from build123d import *

# Parameters (mm, degrees)
BOSS_EXTRUDE1_DEPTH                              = 2.3
BOSS_EXTRUDE2_START                              = 6.7
BOSS_EXTRUDE2_DEPTH                              = 6.7
BOSS_EXTRUDE3_DEPTH                              = 0.5
SKETCH4_R                                        = 12.925
BOSS_EXTRUDE4_DEPTH                              = 7.6
DRAFT1_ANGLE                                     = 56.309932527
DRAFT2_ANGLE                                     = 56.309932527
DRAFT3_ANGLE                                     = 56.309932527
DRAFT4_ANGLE                                     = 56.309932527
SKETCH5_R                                        = 8.025
CUT_EXTRUDE1_DEPTH                               = 8
CUT_EXTRUDE2_DEPTH                               = 1.65
CBORE_FOR_M8_HEX_HEAD_BOLT1_D                    = 9.25
CBORE_FOR_M8_HEX_HEAD_BOLT1_CBORE_D              = 12
CBORE_FOR_M8_HEX_HEAD_BOLT1_CBORE_DEPTH          = 0.65
CBORE_FOR_M3_HEX_HEAD_MACHINE_SCREW1_D           = 3.5
CBORE_FOR_M3_HEX_HEAD_MACHINE_SCREW1_DEPTH       = 9.9
CBORE_FOR_M3_HEX_HEAD_MACHINE_SCREW1_CBORE_D     = 6
CBORE_FOR_M3_HEX_HEAD_MACHINE_SCREW1_CBORE_DEPTH = 2.45
CHAMFER1_SIZE                                    = 0.25
CHAMFER4_SIZE                                    = 0.5
CHAMFER4_SIZE2                                   = 0.9
FILLET1_R                                        = 0.150000001
FILLET2_R                                        = 0.499999999


with BuildPart() as part:
    # Sketch1 → Boss-Extrude1 (new body)
    with BuildSketch(Plane.XZ.offset(-6.7)):
        with BuildLine():
            Line((8.625, -20.875), (16.316766683, -20.875))
            ThreePointArc((16.316766683, -20.875), (17.01460187, -20.749306819), (17.624723932, -20.388026052))
            ThreePointArc((17.624723932, -20.388026052), (19.056527753, -19.056527753), (20.388026052, -17.624723932))
            ThreePointArc((20.388026052, -17.624723932), (20.749306819, -17.01460187), (20.875, -16.316766683))
            Line((20.875, -16.316766683), (20.875, 16.316766683))
            ThreePointArc((20.875, 16.316766683), (20.749306819, 17.01460187), (20.388026052, 17.624723932))
            ThreePointArc((20.388026052, 17.624723932), (19.056527753, 19.056527753), (17.624723932, 20.388026052))
            ThreePointArc((17.624723932, 20.388026052), (17.01460187, 20.749306819), (16.316766683, 20.875))
            Line((16.316766683, 20.875), (-16.316766683, 20.875))
            ThreePointArc((-16.316766683, 20.875), (-17.01460187, 20.749306819), (-17.624723932, 20.388026052))
            ThreePointArc((-17.624723932, 20.388026052), (-19.056527753, 19.056527753), (-20.388026052, 17.624723932))
            ThreePointArc((-20.388026052, 17.624723932), (-20.749306819, 17.01460187), (-20.875, 16.316766683))
            Line((-20.875, 16.316766683), (-20.875, -16.316766683))
            ThreePointArc((-20.875, -16.316766683), (-20.749306819, -17.01460187), (-20.388026052, -17.624723932))
            ThreePointArc((-20.388026052, -17.624723932), (-19.056527753, -19.056527753), (-17.624723932, -20.388026052))
            ThreePointArc((-17.624723932, -20.388026052), (-17.01460187, -20.749306819), (-16.316766683, -20.875))
            Line((-16.316766683, -20.875), (-8.625, -20.875))
            ThreePointArc((-8.625, -20.875), (-8.271446609, -21.02144661), (-8.125, -21.375))
            Line((-8.125, -21.375), (-8.125, -24.875))
            ThreePointArc((-8.125, -24.875), (-8.051776696, -25.051776693), (-7.875000003, -25.124999997))
            Line((-7.875000003, -25.124999997), (7.875000003, -25.124999997))
            ThreePointArc((7.875000003, -25.124999997), (8.051776696, -25.051776693), (8.125, -24.875))
            Line((8.125, -24.875), (8.125, -21.375))
            ThreePointArc((8.125, -21.375), (8.271446609, -21.02144661), (8.625, -20.875))
        make_face()
    extrude(amount=-BOSS_EXTRUDE1_DEPTH)

    # Sketch2 → Boss-Extrude2 (add)
    with BuildSketch(Plane.XZ.offset(-6.7).offset(BOSS_EXTRUDE2_START)):
        with BuildLine():
            Line((-8.2, -19.791378029), (-8.2, -20.875))
            Line((-8.2, -20.875), (-16.316766683, -20.875))
            ThreePointArc((-16.316766683, -20.875), (-17.01460187, -20.749306819), (-17.624723932, -20.388026052))
            ThreePointArc((-17.624723932, -20.388026052), (-19.056527753, -19.056527753), (-20.388026052, -17.624723932))
            ThreePointArc((-20.388026052, -17.624723932), (-20.749306819, -17.01460187), (-20.875, -16.316766683))
            Line((-20.875, -16.316766683), (-20.875, 16.316766683))
            ThreePointArc((-20.875, 16.316766683), (-20.749306819, 17.01460187), (-20.388026052, 17.624723932))
            ThreePointArc((-20.388026052, 17.624723932), (-19.056527753, 19.056527753), (-17.624723932, 20.388026052))
            ThreePointArc((-17.624723932, 20.388026052), (-17.01460187, 20.749306819), (-16.316766683, 20.875))
            Line((-16.316766683, 20.875), (16.316766683, 20.875))
            ThreePointArc((16.316766683, 20.875), (17.01460187, 20.749306819), (17.624723932, 20.388026052))
            ThreePointArc((17.624723932, 20.388026052), (19.056527753, 19.056527753), (20.388026052, 17.624723932))
            ThreePointArc((20.388026052, 17.624723932), (20.749306819, 17.01460187), (20.875, 16.316766683))
            Line((20.875, 16.316766683), (20.875, -16.316766683))
            ThreePointArc((20.875, -16.316766683), (20.749306819, -17.01460187), (20.388026052, -17.624723932))
            ThreePointArc((20.388026052, -17.624723932), (19.056527753, -19.056527753), (17.624723932, -20.388026052))
            ThreePointArc((17.624723932, -20.388026052), (17.01460187, -20.749306819), (16.316766683, -20.875))
            Line((16.316766683, -20.875), (8.199999996, -20.875))
            Line((8.199999996, -20.875), (8.199999996, -19.791378029))
            ThreePointArc((8.199999996, -19.791378029), (8.276120463, -19.408694597), (8.492893215, -19.084271248))
            Line((8.492893215, -19.084271248), (19.207106777, -8.370057685))
            ThreePointArc((19.207106777, -8.370057685), (19.423879528, -8.045634337), (19.499999995, -7.662950906))
            Line((19.499999995, -7.662950906), (19.499999995, 7.662950902))
            ThreePointArc((19.499999995, 7.662950902), (19.423879528, 8.045634333), (19.207106777, 8.370057681))
            Line((19.207106777, 8.370057681), (8.370057681, 19.207106777))
            ThreePointArc((8.370057681, 19.207106777), (8.045634333, 19.423879528), (7.662950902, 19.499999995))
            Line((7.662950902, 19.499999995), (-7.662950906, 19.499999995))
            ThreePointArc((-7.662950906, 19.499999995), (-8.045634337, 19.423879528), (-8.370057685, 19.207106777))
            Line((-8.370057685, 19.207106777), (-19.207106781, 8.370057681))
            ThreePointArc((-19.207106781, 8.370057681), (-19.423879532, 8.045634333), (-19.499999999, 7.662950902))
            Line((-19.499999999, 7.662950902), (-19.499999999, -7.662950906))
            ThreePointArc((-19.499999999, -7.662950906), (-19.423879532, -8.045634337), (-19.207106781, -8.370057685))
            Line((-19.207106781, -8.370057685), (-8.492893219, -19.084271248))
            ThreePointArc((-8.492893219, -19.084271248), (-8.276120467, -19.408694597), (-8.2, -19.791378029))
        make_face()
    extrude(amount=-BOSS_EXTRUDE2_DEPTH)

    # Sketch3 → Boss-Extrude3 (add)
    with BuildSketch(Plane.XZ.offset(-6.7)):
        with BuildLine():
            Line((-11.809681219, -15.767483247), (-15.767483247, -11.809681219))
            ThreePointArc((-15.767483247, -11.809681219), (-12.88370491, -12.88370491), (-11.809681219, -15.767483247))
        make_face()
        with BuildLine():
            Line((-15.767483247, 11.809681219), (-11.809681219, 15.767483247))
            ThreePointArc((-11.809681219, 15.767483247), (-12.88370491, 12.88370491), (-15.767483247, 11.809681219))
        make_face()
        with BuildLine():
            Line((15.767483247, -11.809681219), (11.809681219, -15.767483247))
            ThreePointArc((11.809681219, -15.767483247), (12.88370491, -12.88370491), (15.767483247, -11.809681219))
        make_face()
        with BuildLine():
            Line((11.809681219, 15.767483247), (15.767483247, 11.809681219))
            ThreePointArc((15.767483247, 11.809681219), (12.88370491, 12.88370491), (11.809681219, 15.767483247))
        make_face()
    extrude(amount=BOSS_EXTRUDE3_DEPTH)

    # Sketch4 → Boss-Extrude4 (add)
    with BuildSketch(Plane.XZ.offset(-6.7)):
        with Locations(Location((0, 0, 0), (0, 0, 90))):
            Circle(SKETCH4_R)
    extrude(amount=BOSS_EXTRUDE4_DEPTH)

    # Draft1
    draft1_faces = [part.faces().sort_by_distance(p)[0] for p in [
        (-12.88370491, 6.45, -12.88370491),
    ]]
    draft(draft1_faces, Plane(origin=(-15.5, 6.2, -15.5), x_dir=(0, 0, -1), z_dir=(0, -1, 0)), DRAFT1_ANGLE)

    # Draft2
    draft2_faces = [part.faces().sort_by_distance(p)[0] for p in [
        (-12.88370491, 6.45, 12.88370491),
    ]]
    draft(draft2_faces, Plane(origin=(-15.5, 6.2, 15.5), x_dir=(0, 0, -1), z_dir=(0, -1, 0)), DRAFT2_ANGLE)

    # Draft3
    draft3_faces = [part.faces().sort_by_distance(p)[0] for p in [
        (12.88370491, 6.45, 12.88370491),
    ]]
    draft(draft3_faces, Plane(origin=(15.5, 6.2, 15.5), x_dir=(0, 0, -1), z_dir=(0, -1, 0)), DRAFT3_ANGLE)

    # Draft4
    draft4_faces = [part.faces().sort_by_distance(p)[0] for p in [
        (12.88370491, 6.45, -12.88370491),
    ]]
    draft(draft4_faces, Plane(origin=(15.5, 6.2, -15.5), x_dir=(0, 0, -1), z_dir=(0, -1, 0)), DRAFT4_ANGLE)

    # Sketch5 → Cut-Extrude1 (cut)
    with BuildSketch(Plane.XZ.offset(0.9)):
        with Locations(Location((0, 0, 0), (0, 0, 90))):
            Circle(SKETCH5_R)
    extrude(amount=-CUT_EXTRUDE1_DEPTH, mode=Mode.SUBTRACT)

    # Sketch6 → Cut-Extrude2 (cut)
    with BuildSketch(Plane.XZ.offset(-6.7)):
        with BuildLine():
            Line((6.95, -16.775), (-6.95, -16.775))
            ThreePointArc((-6.95, -16.775), (-7.126776695, -16.848223305), (-7.2, -17.025))
            Line((-7.2, -17.025), (-7.2, -23.925))
            ThreePointArc((-7.2, -23.925), (-7.126776695, -24.101776695), (-6.95, -24.175))
            Line((-6.95, -24.175), (6.95, -24.175))
            ThreePointArc((6.95, -24.175), (7.126776695, -24.101776695), (7.2, -23.925))
            Line((7.2, -23.925), (7.2, -17.025))
            ThreePointArc((7.2, -17.025), (7.126776695, -16.848223305), (6.95, -16.775))
        make_face()
    extrude(amount=-CUT_EXTRUDE2_DEPTH, mode=Mode.SUBTRACT)

    # CBORE for M8 Hex Head Bolt1 (through all)
    with Locations(Plane(origin=(0, 7.1, 0), x_dir=(-1, 0, 0), z_dir=(0, -1, 0))):
        with Locations((0, 0)):
            CounterBoreHole(CBORE_FOR_M8_HEX_HEAD_BOLT1_D / 2, CBORE_FOR_M8_HEX_HEAD_BOLT1_CBORE_D / 2, CBORE_FOR_M8_HEX_HEAD_BOLT1_CBORE_DEPTH)

    # CBORE for M3 Hex Head Machine Screw1
    with Locations(Plane(origin=(0, 9, 0), x_dir=(1, 0, 0), z_dir=(0, 1, 0))):
        with Locations((15.5, 15.5), (15.5, -15.5), (-15.5, 15.5), (-15.5, -15.5)):
            CounterBoreHole(CBORE_FOR_M3_HEX_HEAD_MACHINE_SCREW1_D / 2, CBORE_FOR_M3_HEX_HEAD_MACHINE_SCREW1_CBORE_D / 2, CBORE_FOR_M3_HEX_HEAD_MACHINE_SCREW1_CBORE_DEPTH, depth=CBORE_FOR_M3_HEX_HEAD_MACHINE_SCREW1_DEPTH)

    # Chamfer1
    chamfer1_edges = [part.edges().sort_by_distance(p)[0] for p in [
        (20.749306819, 9, -17.01460187),
        (20.875, 9, 0),
        (20.749306819, 9, 17.01460187),
        (19.056527753, 9, 19.056527753),
        (0, -0.9, -12.925),
        (17.01460187, 9, 20.749306819),
        (6, 7.1, 0),
        (-4.625, 9, 0),
        (0, 9, 20.875),
        (-17.01460187, 9, 20.749306819),
        (-19.056527753, 9, 19.056527753),
        (-20.749306819, 9, 17.01460187),
        (-20.875, 9, 0),
        (17.01460187, 9, -20.749306819),
        (-20.749306819, 9, -17.01460187),
        (-19.056527753, 9, -19.056527753),
        (-17.01460187, 9, -20.749306819),
        (-12.470883342, 9, -20.875),
        (-8.271446609, 9, -21.02144661),
        (-8.125, 9, -23.125),
        (-8.051776696, 9, -25.051776693),
        (0, 9, -25.124999997),
        (8.051776696, 9, -25.051776693),
        (8.125, 9, -23.125),
        (19.056527753, 9, -19.056527753),
        (8.271446609, 9, -21.02144661),
        (12.470883342, 9, -20.875),
    ]]
    chamfer(chamfer1_edges, length=CHAMFER1_SIZE - 0.0001)  # a hair under: the kernel refuses the full size

    # Chamfer4
    chamfer4_edges = [part.edges().sort_by_distance(p)[0] for p in [
        (0, -0.9, -8.025),
    ]]
    chamfer4_side = [part.faces().sort_by_distance(p)[0] for p in [
        (0, -0.9, -12.316594034),
    ]]
    chamfer(chamfer4_edges, length=CHAMFER4_SIZE, length2=CHAMFER4_SIZE2, reference=chamfer4_side[0])

    # Fillet1
    fillet1_edges = [part.edges().sort_by_distance(p)[0] for p in [
        (0, 6.7, -12.925),
    ]]
    fillet(fillet1_edges, radius=FILLET1_R)

    # Fillet2
    fillet2_edges = [part.edges().sort_by_distance(p)[0] for p in [
        (-12.353374823, 6.7, -12.353374823),
        (12.353374823, 6.7, -12.353374823),
        (12.88370491, 6.2, -12.88370491),
    ]]
    fillet(fillet2_edges, radius=FILLET2_R)


solid = part.part
Part model, mm, in its own coordinate system. A direction names the side the tool comes from. Round coordinates to 2 decimals unless told otherwise and drop trailing zeros. Return JSON: item names as keys, results as strings. Group by question number.
(1) Pin check, flat tips, straight feed: pin 1 Ø3 at (x, z) = (-16, -14) entering from +Y; pin 2 Ø5.5 at (x, z) = (15.5, 15.5) entering from -Y; pin 3 Ø3.5 at (x, z) = (-2.5, 0.5) entering from -Y; pin 4 Ø5.5 at (x, z) = (15.5, -15.5) entering from +Y. Stop position of each tip, or through.
(2) Saw through at A-A on y = 5. Count the separate pieces of the cut face and the enclosed holes in it, then the cut area to 3 significant figures.
(3) Which spindle directions (+Z, -Z, +X, -X, +Y, -Y) get a long thin tool onto all of the face, cutting with end or side? Do faces 4 (the face through (17, 6.55, 17)), 5 (the face through (-8.2, 3, -20)), 6 (the face through (-20.75, 4.31, 17.01)), 7 (the face through (-7.2, 8, -20)). Say none if no direction does.
(4) Two-plate mould, pull along X, no slides. Class faces 1 (the face through (-20.875, 4, 0)), 2 (the face through (20.746, 4.314, 17.024)), 3 (the face through (0, 3, 19.5)): +X half, -X half, draft (parallel to the pull), parting line (faces both ways), or undercut.
(5) Drill centre lines: probe 1 along X at (y, z) = (7.4, 15.5) (3 decimals); probe 2 along Z at (x, y) = (0, 7.5) (3 decimals); probe 3 along X at (y, z) = (2, 0) (3 decimals). Where is each one in solid material? Low to high.
Returned:
{
 "1": {"pin 1": "y = 9", "pin 2": "y = 0", "pin 3": "through", "pin 4": "y = 6.55"},
 "2": {"separate pieces": "2", "enclosed holes": "5", "area": "717 mm²"},
 "3": {"face 4": "+Y", "face 5": "-Z, -Y", "face 6": "+Z, -X, +Y, -Y", "face 7": "-Y"},
 "4": {"face 1": "-X half", "face 2": "+X half", "face 3": "undercut"},
 "5": {"probe 1": "-20.875 to -18.5, -12.5 to 12.5, 18.5 to 20.875", "probe 2": "-25.125 to -24.175, -16.775 to -6, 6 to 20.875", "probe 3": "-20.875 to -19.5, -12.925 to -8.025, 8.025 to 12.925, 19.5 to 20.875"}
}
